For this review, take the finished solid that the model builds, in its own axes (mm). A direction names the side the tool comes from. Coordinates: 2 decimals unless noted, no trailing zeros. Loops run counter-clockwise (first coordinate to the right, second up) from the corner with the lowest first, then second, coordinate; pieces in that order, holes last. Notation, with made-up numbers: (-32.75, 62) - (-15.75, 62) arc R18 ccw to (-15.75, 66) - close; hole circle Ø4 at (63.5, 13.5). An arc over 180 degrees is marked (long way). Use one line per item in the form item = value. Start each with the question number.
1. Draft analysis for pull direction Y (two halves, no side actions). For faces 1 (the face through (-1.5, 0.07, 5.32)), 2 (the face through (0, 0, 10.8)), 3 (the face through (0.3, -0.3, 11.3)), state which applies: +Y half, -Y half, draft (parallel to the pull), parting line (faces both ways), or undercut.
2. Add section A-A on z = 2. Give the boundary of the cut face in (x, y).
3. For pin 1 Ø2 at (y, z) = (1, 8.5) entering from +X; pin 2 Ø3 at (x, y) = (1, 1.5) entering from -Z; pin 3 Ø0.6 at (y, z) = (-0.5, 11) entering from -X; pin 4 Ø2 at (x, z) = (-1, 6.5) entering from +Y, all flat-tipped, find the tip position at first contact; note any pin that passes through.
4. Machinability: for faces 4 (the face through (0, -2, 10.8)), 5 (the face through (0, 0, 0)), which of the approach directions +Z, -Z, +X, -X, +Y, -Y give a long, thin tool a straight path to every point of the face, cutting with its end or side? Answer none if there is none.
5. To check wall thickness, follow probe 1 along Y at (x, z) = (-1.1, 11) (3 decimals); probe 2 along Y at (x, z) = (0, 2.5). State the ranges of each line that lie inside material, in increasing order.
```python
from build123d import *

# Parameters (mm, degrees)
F0_R     = 1.5
F1_DEPTH = 11.3
F2_R     = 2.61
F2_R_2   = 1.5
F3_DEPTH = 0.5
F5_DEPTH = 0.5


# Not quite as in the source:
# - a fillet or chamfer that OpenCascade refuses, or shapes differently, is made with other operations: its cross-section is extruded or revolved along the edge and cut away or added


with BuildPart() as f1:
    # F0 (on Top) → F1 (new body)
    with BuildSketch(Plane.XY):
        Circle(F0_R)
    extrude(amount=F1_DEPTH)

    # F2 (on face) → F3 (join)
    with BuildSketch(Plane.XY.offset(11.3)):
        Circle(F2_R)
        Circle(F2_R_2, mode=Mode.SUBTRACT)
    extrude(amount=-F3_DEPTH)

    # F4: fillet of radius 2 on 1 edges, made by hand

    # F4_s1 → F4_t2 (revolve, cut)
    with BuildSketch(Plane.XZ):
        with BuildLine():
            ThreePointArc((2.61, 10.8), (1.9942311257, 11.1708286934), (1.2871243445, 11.3))
            Line((1.2871243445, 11.3), (2.61, 11.3))
            Line((2.61, 11.3), (2.61, 10.8))
        make_face()
    revolve(axis=Axis((0, 0, 11.3), (0, 0, 1)), mode=Mode.SUBTRACT)

    # F2 (on face) → F5 (cut)
    with BuildSketch(Plane.XY.offset(11.3)):
        Polygon((-1.2485300168, 0.125), (-1.2485300168, -0.125), (-0.125, -0.125), (-0.125, -1.2485300168), (0.125, -1.2485300168), (0.125, -0.125), (1.2485300168, -0.125), (1.2485300168, 0.125), (0.125, 0.125), (0.125, 1.2485300168), (-0.125, 1.2485300168), (-0.125, 0.125), align=None)
    extrude(amount=-F5_DEPTH, mode=Mode.SUBTRACT)


solid = f1.part
```
Conclusion:
q1.face_1 = parting line
q1.face_2 = undercut
q1.face_3 = draft
q2.outline = circle Ø3 at (0, 0)
q3.pin_1 = 1.5
q3.pin_2 = 0
q3.pin_3 = -2.6
q3.pin_4 = 1.5
q4.face_4 = -Z
q4.face_5 = -Z, +X, -X, +Y, -Y
q5.probe_1 = -2.066 to -0.125, 0.125 to 2.066
q5.probe_2 = -1.5 to 1.5
